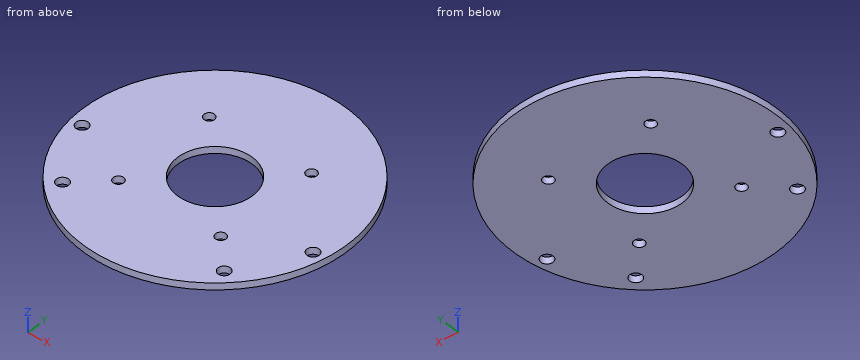
```python
from build123d import *

# Parameters (mm, degrees)
SKETCH_1_R          = 39
EXTRUDE_1_DEPTH     = 2
SKETCH_3_R          = 1.55
CUT_EXTRUDE_2_DEPTH = 2
SKETCH_4_R          = 11.05
CUT_EXTRUDE_3_DEPTH = 2
SKETCH_6_R          = 1.8
CUT_EXTRUDE_4_DEPTH = 10


with BuildPart() as part:
    # 草图1 → 凸台-拉伸1 (new body)
    with BuildSketch(Plane.XY):
        Circle(SKETCH_1_R)
    extrude(amount=EXTRUDE_1_DEPTH)

    # 草图3 → 切除-拉伸2 (cut)
    with BuildSketch(Plane.XY.offset(2)):
        with Locations((-15.5, -15.5)):
            Circle(SKETCH_3_R)
        with Locations((15.5, -15.5)):
            Circle(SKETCH_3_R)
        with Locations((15.5, 15.5)):
            Circle(SKETCH_3_R)
        with Locations((-15.5, 15.5)):
            Circle(SKETCH_3_R)
    extrude(amount=-CUT_EXTRUDE_2_DEPTH, mode=Mode.SUBTRACT)

    # 草图4 → 切除-拉伸3 (cut)
    with BuildSketch(Plane.XY.offset(2)):
        Circle(SKETCH_4_R)
    extrude(amount=-CUT_EXTRUDE_3_DEPTH, mode=Mode.SUBTRACT)

    # 草图6 → 切除-拉伸4 (cut)
    with BuildSketch(Plane.XY.offset(2)):
        with Locations((24.5, -24.459064842)):
            Circle(SKETCH_6_R)
        with Locations((-24.5, -24.459064842)):
            Circle(SKETCH_6_R)
        with Locations((35, -5.959064842)):
            Circle(SKETCH_6_R)
        with Locations((-35, -5.959064842)):
            Circle(SKETCH_6_R)
    extrude(amount=-CUT_EXTRUDE_4_DEPTH, mode=Mode.SUBTRACT)


solid = part.part
```
CAD build for the part. Positions are in the model's coordinates, mm. Round coordinates to 2 decimals unless told otherwise and drop trailing zeros. Write each loop counter-clockwise with the first axis right and the second up, starting at its lowest first coordinate (ties: lowest second). Pieces come first, ordered by that corner, then holes.
Item 1: Band-saw the part on D-D on x = -15.5. Write the cut outline in (y, z), then the cut area to 3 significant figures.
Filled in:
outline: (-35.79, 0) - (-17.05, 0) - (-17.05, 2) - (-35.79, 2) - close; (-13.95, 0) - (13.95, 0) - (13.95, 2) - (-13.95, 2) - close; (17.05, 0) - (35.79, 0) - (35.79, 2) - (17.05, 2) - close
area: 131 mm2
Item 2: Drop flat-ended pins along their axis: pin 1 Ø3 at (x, y) = (-15.5, 15.5) entering from +Z; pin 2 Ø1 at (y, z) = (-30.5, 1) entering from +X. Give the stop position or say it passes through.
Filled in:
pin 1: passes through
pin 2: stops at x = 24.92
Item 3: Band-saw the part on C-C on z = 1.05. Give the number of separate pieces and of enclosed holes in the cut face, then the cut area to 3 significant figures.
Filled in:
separate pieces: 1
enclosed holes: 9
area: 4,320 mm2
Item 4: Band-saw the part on A-A on x = 0. Write the cut outline in (y, z), then the cut area to 3 significant figures.
Filled in:
outline: (-39, 0) - (-11.05, 0) - (-11.05, 2) - (-39, 2) - close; (11.05, 0) - (39, 0) - (39, 2) - (11.05, 2) - close
area: 112 mm2
Item 5: Drill centre lines: L1, parallel to Y at x = -35, z = 0.6; L2, parallel to Y at x = 24.5, z = 1.6; L3, parallel to Y at x = 15, z = 1.7. Where is each one in solid material? Low to high.
Filled in:
L1: y = -17.2 to -7.76, -4.16 to 17.2
L2: y = -30.34 to -26.26, -22.66 to 30.34
L3: y = -36 to -16.97, -14.03 to 14.03, 16.97 to 36
